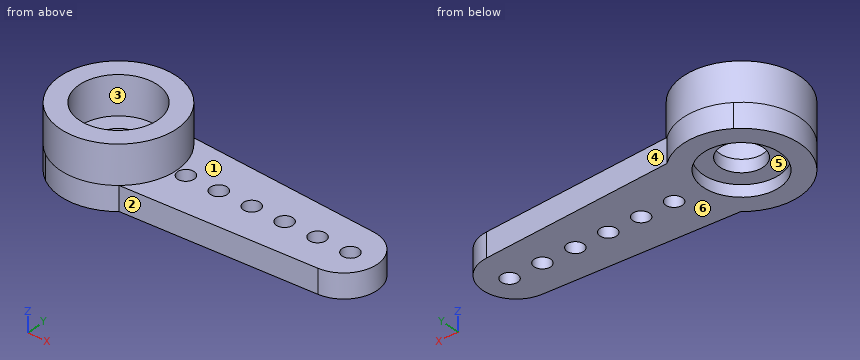
```python
from build123d import *

# Parameters (mm, degrees)
SKETCH_1_R             = 2.775112647
SKETCH_1_R_2           = 2
SKETCH_1_R_3           = 3.5
EXTRUDE_1_DEPTH        = 1.45
SKETCH_2_R             = 3.5
SKETCH_2_R_2           = 2.35
EXTRUDE_2_DEPTH        = 2.3
SKETCH_3_R             = 2.3
CUT_EXTRUDE_1_DEPTH    = 0.7
SKETCH_4_R             = 1.3
CUT_EXTRUDE_2_DEPTH    = 17.372003543
SKETCH_5_R             = 0.5
CUT_EXTRUDE_3_DEPTH    = 17.516733939
PATTERN_LINEAR_1_COUNT = 6
PATTERN_LINEAR_1_PITCH = 2


with BuildPart() as part:
    # 草图1 → 凸台-拉伸1 (new body)
    with BuildSketch(Plane.XY):
        with BuildLine():
            Line((0.157009161, 2.770667488), (-1.972354438, 2.891334981))
            ThreePointArc((-1.972354438, 2.891334981), (-3.5, 0), (-1.972354438, -2.891334981))
            Line((-1.972354438, -2.891334981), (0.1570091, -2.770667491))
            ThreePointArc((0.1570091, -2.770667491), (-2.775112647, 3.1e-08), (0.157009161, 2.770667488))
        make_face()
        with BuildLine():
            Line((2.286372673, 2.65), (0.157009161, 2.770667488))
            ThreePointArc((0.157009161, 2.770667488), (2.017048378, 1.905981649), (2.775112647, 0))
            ThreePointArc((2.775112647, 0), (2.017048356, -1.905981672), (0.1570091, -2.770667491))
            Line((0.1570091, -2.770667491), (2.286372673, -2.65))
            ThreePointArc((2.286372673, -2.65), (3.182161557, -1.457342726), (3.5, 0))
            ThreePointArc((3.5, 0), (3.182161557, 1.457342726), (2.286372673, 2.65))
        make_face()
        Circle(SKETCH_1_R)
        with BuildLine():
            ThreePointArc((2.286372673, 2.65), (0.198021479, 3.494393723), (-1.972354438, 2.891334981))
            Line((-1.972354438, 2.891334981), (0.157009161, 2.770667488))
            Line((0.157009161, 2.770667488), (2.286372673, 2.65))
        make_face()
        with BuildLine():
            Line((0.1570091, -2.770667491), (-1.972354438, -2.891334981))
            ThreePointArc((-1.972354438, -2.891334981), (0.198021479, -3.494393723), (2.286372673, -2.65))
            Line((2.286372673, -2.65), (0.1570091, -2.770667491))
        make_face()
        with BuildLine():
            Line((13.813155138, 1.996796413), (2.286372673, 2.65))
            ThreePointArc((2.286372673, 2.65), (3.182161557, 1.457342726), (3.5, 0))
            ThreePointArc((3.5, 0), (3.182161557, -1.457342726), (2.286372673, -2.65))
            Line((2.286372673, -2.65), (13.813155123, -1.996796414))
            ThreePointArc((13.813155123, -1.996796414), (11.7, 8e-09), (13.813155138, 1.996796413))
        make_face()
        with Locations((13.7, 0)):
            Circle(SKETCH_1_R_2)
        Circle(SKETCH_1_R_3)
    extrude(amount=EXTRUDE_1_DEPTH)

    # 草图2 → 凸台-拉伸2 (add)
    with BuildSketch(Plane.XY.offset(1.45)):
        with Locations(Location((0, 0, 0), (0, 0, 310.787038193))):
            Circle(SKETCH_2_R)
        Circle(SKETCH_2_R_2, mode=Mode.SUBTRACT)
    extrude(amount=EXTRUDE_2_DEPTH)

    # 草图3 → 切除-拉伸1 (cut)
    with BuildSketch(Plane(origin=(0, 0, 0), x_dir=(-1, 0, 0), z_dir=(0, 0, -1))):
        Circle(SKETCH_3_R)
    extrude(amount=-CUT_EXTRUDE_1_DEPTH, mode=Mode.SUBTRACT)

    # 草图4 → 切除-拉伸2 (cut, through all)
    with BuildSketch(Plane(origin=(0, 0, 0.7), x_dir=(-1, 0, 0), z_dir=(0, 0, -1))):
        Circle(SKETCH_4_R)
    extrude(amount=-CUT_EXTRUDE_2_DEPTH, mode=Mode.SUBTRACT)

    # 草图5 → 切除-拉伸3 (cut, through all)
    with BuildSketch(Plane(origin=(0, 0, 0), x_dir=(-1, 0, 0), z_dir=(0, 0, -1))):
        with Locations((-14.1, 0)):
            Circle(SKETCH_5_R)
    cut_extrude_3 = extrude(amount=-CUT_EXTRUDE_3_DEPTH, mode=Mode.SUBTRACT)

    # 阵列(线性)1: 切除-拉伸3 ×6
    with Locations(*[(-i * PATTERN_LINEAR_1_PITCH, 0, 0) for i in range(1, PATTERN_LINEAR_1_COUNT)]):
        add(cut_extrude_3, mode=Mode.SUBTRACT)


solid = part.part
```
CAD build for the part. Positions are in the model's coordinates, mm. Face numbers are marked on the shaded views. A direction names the side the tool comes from. Round coordinates to 2 decimals unless told otherwise and drop trailing zeros. Write each loop counter-clockwise with the first axis right and the second up, starting at its lowest first coordinate (ties: lowest second). Pieces come first, ordered by that corner, then holes. Notation, with made-up numbers: (54.25, 66) - (99.25, 66) arc R12 cw to (99.25, 82) - close; hole circle Ø10 at (-4.5, 51). An arc over 180 degrees is marked (long way). Write item = value, one per line. Start each with the question number.
Q1. Probe L1, parallel to Y at x = 0, z = 2.9; L2, parallel to Z at x = 0.25, y = -1.5; L3, parallel to Z at x = 14.5, y = -0.5. List the from-to ranges inside material, lowest first. Write a range as from..to.
Q2. Band-saw the part on C-C (x = 0.75). Give the cut face in (y, z).
Q3. Mould opens along Y. For the marked faces 1, 2, 3 and 4 say: pulls with the +Y half, pulls with the -Y half, needs draft (parallel to the pull), parting line crosses it, or undercut.
Q4. Drop flat-ended pins along their axis: pin 1 (2 mm diameter, centred on y = -2, z = 2, fed in from -X); pin 2 (1.4 mm diameter, centred on x = -0.5, y = -1, fed in from +Z); pin 3 (2 mm diameter, centred on x = 0, y = 0, fed in from +Z); pin 4 (2 mm diameter, centred on x = 2, z = 1.5, fed in from -Y). Give the stop position or say it passes through.
Q5. Band-saw the part on D-D (z = 2.3). Give the cut face in (x, y), then the cut area to 3 significant figures.
Q6. Band-saw the part on B-B (y = 0.75). Give the cut face in (x, z), then the cut area to 3 significant figures.
Q7. Band-saw the part on A-A (x = 10.1). Give the cut face in (y, z), then the cut area to 3 significant figures.
Q8. Which spindle directions (+Z, -Z, +X, -X, +Y, -Y) get a long thin tool onto all of the face, cutting with end or side? Do the marked faces 5 and 6. Say none if no direction does.
Answers below:
q1.L1 = -3.5..-2.35, 2.35..3.5
q1.L2 = 0.7..1.45
q1.L3 = 0..1.45
q2.outline = (-3.42, 0) - (-2.17, 0) - (-2.17, 0.7) - (-1.06, 0.7) - (-1.06, 1.45) - (-2.23, 1.45) - (-2.23, 3.75) - (-3.42, 3.75) - close; (1.06, 0.7) - (2.17, 0.7) - (2.17, 0) - (3.42, 0) - (3.42, 3.75) - (2.23, 3.75) - (2.23, 1.45) - (1.06, 1.45) - close
q3.face_1 = needs draft
q3.face_2 = pulls with the -Y half
q3.face_3 = undercut
q3.face_4 = pulls with the +Y half
q4.pin_1 = -3.35
q4.pin_2 = 1.45
q4.pin_3 = through
q4.pin_4 = -3.35
q5.outline = circle Ø7 at (0, 0); hole circle Ø4.7 at (0, 0)
q5.area = 21.1 mm2
q6.outline = (-3.42, 0) - (-2.17, 0) - (-2.17, 0.7) - (-1.06, 0.7) - (-1.06, 1.45) - (-2.23, 1.45) - (-2.23, 3.75) - (-3.42, 3.75) - close; (1.06, 0.7) - (2.17, 0.7) - (2.17, 0) - (15.55, 0) - (15.55, 1.45) - (3.42, 1.45) - (3.42, 3.75) - (2.23, 3.75) - (2.23, 1.45) - (1.06, 1.45) - close
q6.area = 28.4 mm2
q7.outline = (-2.21, 0) - (-0.5, 0) - (-0.5, 1.45) - (-2.21, 1.45) - close; (0.5, 0) - (2.21, 0) - (2.21, 1.45) - (0.5, 1.45) - close
q7.area = 4.95 mm2
q8.face_5 = -Z
q8.face_6 = -Z, +X, -X, +Y, -Y
